Verification items for the finished model (mm, model axes). Face numbers are marked on the shaded views. A direction names the side the tool comes from. Coordinates: 2 decimals unless noted, no trailing zeros. Order: outer loops, then holes, each group sorted by start corner. A loop starts at its lowest first (then second) coordinate and runs counter-clockwise, first axis right, second up. Notation, with made-up numbers: M 31.25,-27 L 85.25,-27 A5 cw 85.25,-20 Z; hole C 7.5,-32.75 d1. An arc over 180 degrees is marked long. Return JSON: item names as keys, results as strings.
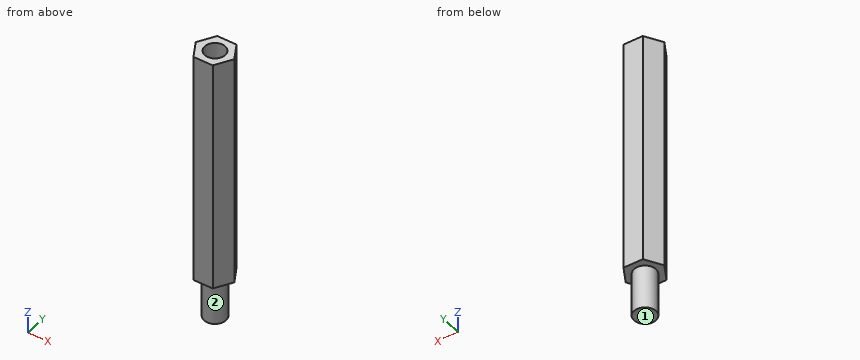
```python
from build123d import *

# Parameters (mm, degrees)
SKETCH_1_R      = 1.4
EXTRUDE_1_DEPTH = 32
SKETCH_2_R      = 1.5
EXTRUDE_2_DEPTH = 6


with BuildPart() as part:
    # 草图1 → 凸台-拉伸1 (new body)
    with BuildSketch(Plane.XY):
        Polygon((2.655811238, 0), (1.327905619, 2.3), (-1.327905619, 2.3), (-2.655811238, 0), (-1.327905619, -2.3), (1.327905619, -2.3), align=None)
        Circle(SKETCH_1_R, mode=Mode.SUBTRACT)
    extrude(amount=EXTRUDE_1_DEPTH)

    # 草图2 → 凸台-拉伸2 (add)
    with BuildSketch(Plane(origin=(0, 0, 0), x_dir=(-1, 0, 0), z_dir=(0, 0, -1))):
        Circle(SKETCH_2_R)
    extrude(amount=EXTRUDE_2_DEPTH)


solid = part.part
```
Q1. Cross-section at A-A, the plane z = 21. Record the boundary of the cut face in (x, y), and give its area (3 significant figures).
Values:
{"outline": "M -2.66,0 L -1.33,-2.3 L 1.33,-2.3 L 2.66,0 L 1.33,2.3 L -1.33,2.3 Z; hole C 0,0 d2.8", "area": "12.2 mm^2"}
Q2. Cross-section at B-B, the plane x = 0. Record the boundary of the cut face in (y, z), and give its area (3 significant figures).
Values:
{"outline": "M -2.3,0 L -1.5,0 L -1.5,-6 L 1.5,-6 L 1.5,0 L 2.3,0 L 2.3,32 L 1.4,32 L 1.4,0 L -1.4,0 L -1.4,32 L -2.3,32 Z", "area": "75.6 mm^2"}
Q3. Tool access check on the marked faces 1 and 2. Record the directions out of +Z, -Z, +X, -X, +Y, -Y that give a thin tool (end or side, any length) a straight path to the whole face; none if there is none.
Values:
{"face 1": "-Z, +X, -X, +Y, -Y", "face 2": "-Z"}
Q4. Material ranges on line 1 along Y through (x, z) = (0, 25); line 2 along Z through (x, y) = (-1.8, 0); line 3 along X through (y, z) = (2, 22), recorded low to high.
Values:
{"line 1": "-2.3 to -1.4, 1.4 to 2.3", "line 2": "0 to 32", "line 3": "-1.5 to 1.5"}
Q5. Cross-section at C-C, the plane z = -3. Record the boundary of the cut face in (x, y), and give its area (3 significant figures).
Values:
{"outline": "C 0,0 d3", "area": "7.07 mm^2"}
Q6. Cross-section at D-D, the plane x = 1.9. Record the boundary of the cut face in (y, z), and give its area (3 significant figures).
Values:
{"outline": "M -1.31,0 L 1.31,0 L 1.31,32 L -1.31,32 Z", "area": "83.8 mm^2"}
